```python
from build123d import *

# Parameters (mm, degrees)
BOSS_EXTRUDE1_DEPTH = 15
SKETCH2_W           = 55
SKETCH2_H           = 34
CUT_EXTRUDE1_DEPTH  = 12
CUT_EXTRUDE2_REACH  = 72
SKETCH4_R           = 1.6
CUT_EXTRUDE3_DEPTH  = 4
BOSS_EXTRUDE3_REACH = 17
SKETCH7_R           = 1.45
CUT_EXTRUDE4_DEPTH  = 16
SKETCH8_R           = 3
CUT_EXTRUDE5_DEPTH  = 4


with BuildPart() as part:
    # Sketch1 → Boss-Extrude1 (new body)
    with BuildSketch(Plane(origin=(0, 0, 0), x_dir=(1, 0, 0), z_dir=(0, 1, 0))):
        with BuildLine():
            Line((35, 20), (35, 7))
            ThreePointArc((35, 7), (28, 0), (35, -7))
            Line((35, -7), (35, -20))
            Line((35, -20), (-35, -20))
            Line((-35, -20), (-35, 20))
            Line((-35, 20), (35, 20))
        make_face()
    extrude(amount=BOSS_EXTRUDE1_DEPTH)

    # Sketch2 → Cut-Extrude1 (cut)
    with BuildSketch(Plane(origin=(0, 15, 0), x_dir=(1, 0, 0), z_dir=(0, 1, 0))):
        with Locations((-4.5, 0)):
            Rectangle(SKETCH2_W, SKETCH2_H)
    extrude(amount=-CUT_EXTRUDE1_DEPTH, mode=Mode.SUBTRACT)

    # Sketch4 → Cut-Extrude2 (cut, up to next)
    with BuildSketch(Plane(origin=(35, 0, 0), x_dir=(0, 0, -1), z_dir=(1, 0, 0)), mode=Mode.PRIVATE) as cut_extrude2_sk1:
        with Locations((11, 7.5)):
            Circle(SKETCH4_R)
    cut_extrude2_tool1 = extrude(cut_extrude2_sk1.sketch, amount=-CUT_EXTRUDE2_REACH, mode=Mode.PRIVATE) & part.part
    add(cut_extrude2_tool1.solids().sort_by_distance((35, 7.5, -11))[0], mode=Mode.SUBTRACT)
    # Sketch4 → Cut-Extrude2 (cut, up to next)
    with BuildSketch(Plane(origin=(35, 0, 0), x_dir=(0, 0, -1), z_dir=(1, 0, 0)), mode=Mode.PRIVATE) as cut_extrude2_sk2:
        with Locations((-11, 7.5)):
            Circle(SKETCH4_R)
    cut_extrude2_tool2 = extrude(cut_extrude2_sk2.sketch, amount=-CUT_EXTRUDE2_REACH, mode=Mode.PRIVATE) & part.part
    add(cut_extrude2_tool2.solids().sort_by_distance((35, 7.5, 11))[0], mode=Mode.SUBTRACT)

    # Sketch5 → Cut-Extrude3 (cut)
    with BuildSketch(Plane.ZY.offset(-23)):
        Polygon((-11, 10.75), (-13.814582562, 9.125), (-13.814582562, 5.875), (-11, 4.25), (-8.185417438, 5.875), (-8.185417438, 9.125), align=None)
        Polygon((8.185417438, 9.125), (8.185417438, 5.875), (11, 4.25), (13.814582562, 5.875), (13.814582562, 9.125), (11, 10.75), align=None)
    extrude(amount=-CUT_EXTRUDE3_DEPTH, mode=Mode.SUBTRACT)

    # Sketch6 → Boss-Extrude3 (add, up to next)
    with BuildSketch(Plane(origin=(0, 15, 0), x_dir=(1, 0, 0), z_dir=(0, 1, 0)), mode=Mode.PRIVATE) as boss_extrude3_sk1:
        with BuildLine():
            Line((-32, -14), (-32, -17))
            Line((-32, -17), (-29, -17))
            ThreePointArc((-29, -17), (-29.878679656, -14.878679656), (-32, -14))
        make_face()
    boss_extrude3_tool1 = extrude(boss_extrude3_sk1.sketch, amount=-BOSS_EXTRUDE3_REACH, mode=Mode.PRIVATE) - part.part
    add(boss_extrude3_tool1.solids().sort_by_distance((-30.72676, 15, 15.72676))[0])
    # Sketch6 → Boss-Extrude3 (add, up to next)
    with BuildSketch(Plane(origin=(0, 15, 0), x_dir=(1, 0, 0), z_dir=(0, 1, 0)), mode=Mode.PRIVATE) as boss_extrude3_sk2:
        with BuildLine():
            Line((23, -14), (23, -17))
            Line((23, -17), (20, -17))
            ThreePointArc((20, -17), (20.878679656, -14.878679656), (23, -14))
        make_face()
    boss_extrude3_tool2 = extrude(boss_extrude3_sk2.sketch, amount=-BOSS_EXTRUDE3_REACH, mode=Mode.PRIVATE) - part.part
    add(boss_extrude3_tool2.solids().sort_by_distance((21.72676, 15, 15.72676))[0])
    # Sketch6 → Boss-Extrude3 (add, up to next)
    with BuildSketch(Plane(origin=(0, 15, 0), x_dir=(1, 0, 0), z_dir=(0, 1, 0)), mode=Mode.PRIVATE) as boss_extrude3_sk3:
        with BuildLine():
            Line((20, 17), (23, 17))
            Line((23, 17), (23, 14))
            ThreePointArc((23, 14), (20.878679656, 14.878679656), (20, 17))
        make_face()
    boss_extrude3_tool3 = extrude(boss_extrude3_sk3.sketch, amount=-BOSS_EXTRUDE3_REACH, mode=Mode.PRIVATE) - part.part
    add(boss_extrude3_tool3.solids().sort_by_distance((21.72676, 15, -15.72676))[0])
    # Sketch6 → Boss-Extrude3 (add, up to next)
    with BuildSketch(Plane(origin=(0, 15, 0), x_dir=(1, 0, 0), z_dir=(0, 1, 0)), mode=Mode.PRIVATE) as boss_extrude3_sk4:
        with BuildLine():
            Line((-32, 14), (-32, 17))
            Line((-32, 17), (-29, 17))
            ThreePointArc((-29, 17), (-29.878679656, 14.878679656), (-32, 14))
        make_face()
    boss_extrude3_tool4 = extrude(boss_extrude3_sk4.sketch, amount=-BOSS_EXTRUDE3_REACH, mode=Mode.PRIVATE) - part.part
    add(boss_extrude3_tool4.solids().sort_by_distance((-30.72676, 15, -15.72676))[0])

    # Sketch7 → Cut-Extrude4 (cut, through all)
    with BuildSketch(Plane(origin=(0, 15, 0), x_dir=(1, 0, 0), z_dir=(0, 1, 0))):
        with Locations((-32, 17)):
            Circle(SKETCH7_R)
        with Locations((23, 17)):
            Circle(SKETCH7_R)
        with Locations((23, -17)):
            Circle(SKETCH7_R)
        with Locations((-32, -17)):
            Circle(SKETCH7_R)
    extrude(amount=-CUT_EXTRUDE4_DEPTH, mode=Mode.SUBTRACT)

    # Sketch8 → Cut-Extrude5 (cut, through all)
    with BuildSketch(Plane.XY.offset(-17)):
        with Locations((-6, 9)):
            Circle(SKETCH8_R)
    extrude(amount=-CUT_EXTRUDE5_DEPTH, mode=Mode.SUBTRACT)


solid = part.part
```
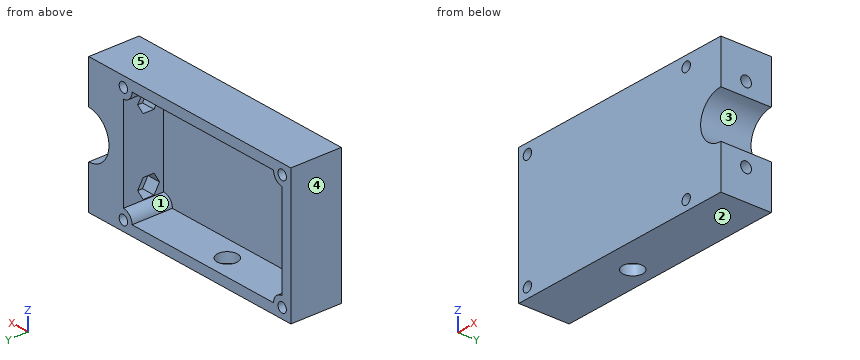
Could you check a few things on this model? Use its own coordinates, in mm. Face numbers are marked on the shaded views. A direction names the side the tool comes from. Round coordinates to 2 decimals unless told otherwise and drop trailing zeros. Loops run counter-clockwise (first coordinate to the right, second up) from the corner with the lowest first, then second, coordinate; pieces in that order, holes last. Notation, with made-up numbers: M 10.5,-17 L 24.5,-17 A25 ccw 24.5,1 Z; hole C 79,59 d5. An arc over 180 degrees is marked long. Write item = value, one per line.
1. I want a section at A-A, the plane x = -6. Write out the boundary of the cut face in (y, z).
Results below:
outline = M 0,-20 L 6,-20 L 6,-17 L 3,-17 L 3,17 L 15,17 L 15,20 L 0,20 Z; M 12,-20 L 15,-20 L 15,-17 L 12,-17 Z
2. I need wall thicknesses on probe 1 along X at (y, z) = (8, 9); probe 2 along X at (y, z) = (13.5, 7.5); probe 3 along Z at (x, y) = (-13, 11.5). Which ranges of each line are inside material? Lowest first, please.
Results below:
probe_1 = -35 to -32, 27 to 35
probe_2 = -35 to -32, 23 to 35
probe_3 = -20 to -17, 17 to 20
3. Thinking about a two-plate mould opening in Z: for the marked faces 3, 4 and 5, which applies, +Z half, -Z half, draft (parallel to the pull), parting line (faces both ways), or undercut?
Results below:
face_3 = undercut
face_4 = draft
face_5 = +Z half
4. Will these pins go through, and if not, where does the flat tip stop? P1, Ø6, axis at y = 10, z = -4.5, coming from the +X side; P2, Ø17, axis at x = -11, z = -3, coming from the +Y side; P3, Ø2.5, axis at x = 23, z = -17, coming from the -Y side.
Results below:
P1 = 35
P2 = 3
P3 = through
5. Which directions (+Z, -Z, +X, -X, +Y, -Y) give clear straight access to the entire face, cutting with the end or side of a thin tool? Please do the marked faces 1 and 2.
Results below:
face_1 = +Y
face_2 = -Z, +X, -X, +Y, -Y
6. I want a section at B-B, the plane y = 13.5. Write out the boundary of the cut face in (x, z).
Results below:
outline = M -35,-20 L 35,-20 L 35,-7 A7 cw 35,7 L 35,20 L -35,20 Z; hole C -32,-17 d2.9; hole C -32,17 d2.9; hole M -32,-14 A3 cw -29,-17 L 20,-17 A3 cw 23,-14 L 23,14 A3 cw 20,17 L -29,17 A3 cw -32,14 Z; hole C 23,-17 d2.9; hole C 23,17 d2.9
7. I want a section at D-D, the plane y = 8.25. Count the separate pieces of the cut face and the enclosed holes in it, and give its area (3 significant figures).
Results below:
separate_pieces = 3
enclosed_holes = 4
area = 747 mm²
8. I want a section at C-C, the plane z = 0. Write out the boundary of the cut face in (x, y), and give its area (3 significant figures).
Results below:
outline = M -35,0 L 28,0 L 28,15 L 23,15 L 23,3 L -32,3 L -32,15 L -35,15 Z
area = 285 mm²
